Design review of the part built by this model. Coordinates are the model's own, in mm. Face numbers are marked on the shaded views. A direction names the side the tool comes from. Give positions to 0.01 mm unless a question says otherwise; leave off trailing zeros. Loops run counter-clockwise (first coordinate to the right, second up) from the corner with the lowest first, then second, coordinate; pieces in that order, holes last. Notation, with made-up numbers: (39, 69.5) -> (75, 69.5) arc R33 ccw to (75, 102.5) -> close; hole circle Ø11 at (39.5, -37.5). An arc over 180 degrees is marked (long way). Answer in a Markdown table with one row per item. Add a question column.
(1) For the marked faces 4 and 5, list the 3-axis set-ups (+Z, -Z, +X, -X, +Y, -Y) from which the entire face can be reached by the end or side of a thin tool; tool diameter is ignored.
(2) Consider section A-A on x = -12.5. Write out the cut boundary in (y, z).
(3) For line 1 (X direction, y = -22, z = 1.5); line 2 (X direction, y = -1.5, z = 0.5); line 3 (X direction, y = -5, z = 5.25), list the stretches that pass through material, from the lowest coordinate up.
(4) For pin 1 (1.5 mm diameter, centred on x = 15, y = -23.5, fed in from +Z), flat-tipped, find the tip position at first contact; note if it passes through.
(5) Consider section C-C on x = 18. Write out the cut boundary in (y, z), then the cut area to 3 significant figures.
(6) Consider section B-B on y = -38.5. Write out the cut boundary in (x, z).
(7) Draft analysis for pull direction X (two halves, no side actions). For the marked faces 1, 2 and 3, state which applies: +X half, -X half, draft (parallel to the pull), parting line (faces both ways), or undercut.
(8) Consider section D-D on y = -1.5. Write out the cut boundary in (x, z), then the cut area to 3 significant figures.
from build123d import *

# Parameters (mm, degrees)
F1_DEPTH = 6.35


with BuildPart() as f1:
    # F0 (on Top) → F1 (new body)
    with BuildSketch(Plane.XY):
        with BuildLine():
            ThreePointArc((0.454082, 0.478478), (0.278106, 0.901741), (-0.146081, 1.07548))
            Line((-0.146081, 1.07548), (0, -26.589924))
            Line((0, -26.589924), (2.290883, -16.137376))
            Line((2.290883, -16.137376), (5.173199, -13.055723))
            ThreePointArc((5.173199, -13.055723), (4.397622, -11.688582), (3.744518, -10.25888))
            ThreePointArc((3.744518, -10.25888), (4.023673, -9.383817), (4.648638, -8.710705))
            ThreePointArc((4.648638, -8.710705), (4.716945, -8.66563), (4.78695, -8.623243))
            Line((4.78695, -8.623243), (5.040929, -8.46264))
            ThreePointArc((5.040929, -8.46264), (10.876438, -4.374773), (16.930446, -0.618068))
            ThreePointArc((16.930446, -0.618068), (22.537122, -7.43494), (22.926339, -16.252709))
            ThreePointArc((22.926339, -16.252709), (14.785708, -17.964937), (6.485587, -17.408523))
            ThreePointArc((6.485587, -17.408523), (10.444862, -23.908384), (13.347887, -30.943759))
            ThreePointArc((13.347887, -30.943759), (11.104788, -36.022973), (6.854687, -39.596003))
            ThreePointArc((6.854687, -39.596003), (5.992693, -35.201596), (6.407121, -30.742662))
            ThreePointArc((6.407121, -30.742662), (8.702961, -30.642489), (8.737067, -32.94026))
            ThreePointArc((8.737067, -32.94026), (8.317875, -29.25748), (4.921873, -30.742662))
            ThreePointArc((4.921873, -30.742662), (4.494337, -36.621274), (6.854687, -42.022163))
            ThreePointArc((6.854687, -42.022163), (12.773811, -37.539563), (16.183371, -30.943759))
            ThreePointArc((16.183371, -30.943759), (14.258029, -25.726553), (11.451863, -20.925343))
            ThreePointArc((11.451863, -20.925343), (18.414863, -20.703369), (25.22471, -19.234144))
            ThreePointArc((25.22471, -19.234144), (25.555314, -6.440003), (16.92072, 3.006856))
            ThreePointArc((16.92072, 3.006856), (10.098074, -1.120915), (3.539007, -5.655849))
            ThreePointArc((3.539007, -5.655849), (3.019272, -5.73262), (2.542413, -5.512112))
            ThreePointArc((2.542413, -5.512112), (2.439849, -4.073337), (2.453046, -2.630971))
            ThreePointArc((2.453046, -2.630971), (2.454254, -2.606818), (2.455495, -2.582667))
            ThreePointArc((2.455495, -2.582667), (1.977854, -2.105025), (1.500212, -2.582667))
            ThreePointArc((1.500212, -2.582667), (1.516702, -3.568582), (1.197531, -4.50155))
            ThreePointArc((1.197531, -4.50155), (0.94141, -4.757671), (0.685288, -4.50155))
            ThreePointArc((0.685288, -4.50155), (0.126595, -2.032107), (0.454082, 0.478478))
        make_face()
        with BuildLine():
            ThreePointArc((1.165291, -14.479887), (0.526476, -14.196909), (0.752014, -13.535627))
            Line((0.752014, -13.535627), (2.261646, -12.653382))
            ThreePointArc((2.261646, -12.653382), (2.970165, -12.840341), (2.781119, -13.548306))
            Line((2.781119, -13.548306), (1.165291, -14.479887))
        make_face(mode=Mode.SUBTRACT)
        with BuildLine():
            Line((0, -26.589924), (-0.146081, 1.07548))
            ThreePointArc((-0.146081, 1.07548), (-0.568409, 0.897272), (-0.739906, 0.472174))
            ThreePointArc((-0.739906, 0.472174), (-0.385925, -2.034813), (-0.918509, -4.510018))
            ThreePointArc((-0.918509, -4.510018), (-1.171911, -4.76883), (-1.430723, -4.515428))
            ThreePointArc((-1.430723, -4.515428), (-1.759729, -3.585882), (-1.753651, -2.599848))
            ThreePointArc((-1.753651, -2.599848), (-2.23631, -2.127277), (-2.708881, -2.609936))
            ThreePointArc((-2.708881, -2.609936), (-2.707385, -2.634073), (-2.705922, -2.658212))
            ThreePointArc((-2.705922, -2.658212), (-2.677494, -4.100358), (-2.764858, -5.540136))
            ThreePointArc((-2.764858, -5.540136), (-3.239361, -5.765667), (-3.759878, -5.694389))
            ThreePointArc((-3.759878, -5.694389), (-10.36647, -1.228974), (-17.232326, 2.826518))
            ThreePointArc((-17.232326, 2.826518), (-25.766677, -6.710997), (-25.300982, -19.500933))
            ThreePointArc((-25.300982, -19.500933), (-18.475999, -20.898162), (-11.511044, -21.046594))
            ThreePointArc((-11.511044, -21.046594), (-14.266352, -25.877169), (-16.136491, -31.114416))
            ThreePointArc((-16.136491, -31.114416), (-12.657468, -37.673847), (-6.691336, -42.09369))
            ThreePointArc((-6.691336, -42.09369), (-4.388153, -36.668176), (-4.877745, -30.794407))
            ThreePointArc((-4.877745, -30.794407), (-8.289241, -29.34517), (-8.669519, -33.032172))
            ThreePointArc((-8.669519, -33.032172), (-8.659679, -30.734169), (-6.36291, -30.810091))
            ThreePointArc((-6.36291, -30.810091), (-5.901417, -35.2644), (-6.716957, -39.667664))
            ThreePointArc((-6.716957, -39.667664), (-11.004554, -36.139716), (-13.301165, -31.084473))
            ThreePointArc((-13.301165, -31.084473), (-10.472597, -24.018834), (-6.582184, -17.477524))
            ThreePointArc((-6.582184, -17.477524), (-14.875966, -18.121559), (-23.034224, -16.495393))
            ThreePointArc((-23.034224, -16.495393), (-22.738146, -7.674005), (-17.20377, -0.798306))
            ThreePointArc((-17.20377, -0.798306), (-11.110429, -4.490869), (-5.232076, -8.516884))
            Line((-5.232076, -8.516884), (-4.976416, -8.674796))
            ThreePointArc((-4.976416, -8.674796), (-4.905966, -8.716442), (-4.837188, -8.760792))
            ThreePointArc((-4.837188, -8.760792), (-4.20515, -9.427268), (-3.916769, -10.299333))
            ThreePointArc((-3.916769, -10.299333), (-4.554739, -11.735853), (-5.315835, -13.111108))
            Line((-5.315835, -13.111108), (-2.401136, -16.162151))
            Line((-2.401136, -16.162151), (0, -26.589924))
        make_face()
        with BuildLine():
            Line((-2.408693, -12.678042), (-0.889828, -13.544297))
            ThreePointArc((-0.889828, -13.544297), (-0.657319, -14.20316), (-1.293111, -14.492868))
            Line((-1.293111, -14.492868), (-2.918687, -13.578403))
            ThreePointArc((-2.918687, -13.578403), (-3.115198, -12.872473), (-2.408693, -12.678042))
        make_face(mode=Mode.SUBTRACT)
    extrude(amount=F1_DEPTH)


solid = f1.part
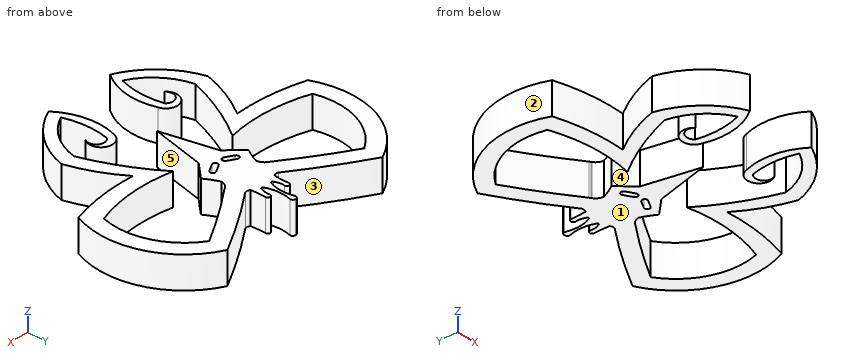
Values follow:
| question | item | result |
|---|---|---|
| 1 | face 4 | +Z, -Z |
| 1 | face 5 | +Z, -Z, -Y |
| 2 | outline | (-37.85, 0) -> (-33.61, 0) -> (-33.61, 6.35) -> (-37.85, 6.35) -> close; (-28.73, 0) -> (-22.56, 0) -> (-22.56, 6.35) -> (-28.73, 6.35) -> close; (-21.1, 0) -> (-18.17, 0) -> (-18.17, 6.35) -> (-21.1, 6.35) -> close; (-3.61, 0) -> (0.09, 0) -> (0.09, 6.35) -> (-3.61, 6.35) -> close |
| 3 | line 1 | -12.15 to -9.42, -1.06 to 1.01, 9.42 to 12.18 |
| 3 | line 2 | -22.76 to -18.2, -15.99 to -9.94, -0.39 to 0.12, 9.52 to 15.44, 18.18 to 22.69 |
| 3 | line 3 | -25.04 to -21.4, -10.33 to -4.73, -2.72 to 2.49, 4.44 to 9.94, 21.32 to 24.94 |
| 4 | pin 1 | through |
| 5 | outline | (-20.75, 0) -> (-17.57, 0) -> (-17.57, 6.35) -> (-20.75, 6.35) -> close; (-1.36, 0) -> (2.44, 0) -> (2.44, 6.35) -> (-1.36, 6.35) -> close |
| 5 | area | 44.4 mm2 |
| 6 | outline | (-11.9, 0) -> (-8.62, 0) -> (-8.62, 6.35) -> (-11.9, 6.35) -> close; (-6.37, 0) -> (-4.83, 0) -> (-4.83, 6.35) -> (-6.37, 6.35) -> close; (4.97, 0) -> (6.52, 0) -> (6.52, 6.35) -> (4.97, 6.35) -> close; (8.62, 0) -> (11.9, 0) -> (11.9, 6.35) -> (8.62, 6.35) -> close |
| 7 | face 1 | draft |
| 7 | face 2 | -X half |
| 7 | face 3 | undercut |
| 8 | outline | (-22.76, 0) -> (-18.2, 0) -> (-18.2, 6.35) -> (-22.76, 6.35) -> close; (-15.99, 0) -> (-9.94, 0) -> (-9.94, 6.35) -> (-15.99, 6.35) -> close; (-0.39, 0) -> (0.12, 0) -> (0.12, 6.35) -> (-0.39, 6.35) -> close; (9.52, 0) -> (15.44, 0) -> (15.44, 6.35) -> (9.52, 6.35) -> close; (18.18, 0) -> (22.69, 0) -> (22.69, 6.35) -> (18.18, 6.35) -> close |
| 8 | area | 137 mm2 |
